from build123d import *

# Parameters (mm, degrees)
SKETCH1_W              = 22.27
SKETCH1_H              = 37
BOSS_EXTRUDE1_DEPTH    = 60
SHELL1_T               = -1
CONVERT_SOLID1_DEPTH   = 60
CONVERT_SOLID1_2_DEPTH = 60
SKETCH6_R              = 2.25
CUT_EXTRUDE1_DEPTH     = 72.365175156


# Read off the part's stored shape, not the designer's step: Convert-Solid1
with BuildPart() as part:
    # Sketch1 → Boss-Extrude1 (new body)
    with BuildSketch(Plane.XY):
        Rectangle(SKETCH1_W, SKETCH1_H)
    extrude(amount=BOSS_EXTRUDE1_DEPTH)

    # Shell1
    shell1_openings = [part.faces().sort_by_distance(p)[0] for p in [
        (0, 0, 60),
        (0, 0, 0),
        (11.135, 0, 30),
    ]]
    offset(amount=SHELL1_T, openings=shell1_openings, kind=Kind.INTERSECTION)

    # Convert-Solid1 outline → Convert-Solid1 (cut)
    with BuildSketch(Plane.XY):
        with BuildLine():
            Line((-11.135, 18.5), (-11.135, 16.23))
            ThreePointArc((-11.135, 16.23), (-10.470132393, 17.835132393), (-8.865, 18.5))
            Line((-8.865, 18.5), (-11.135, 18.5))
        make_face()
        with BuildLine():
            ThreePointArc((-8.865, -18.5), (-10.470132393, -17.835132393), (-11.135, -16.23))
            Line((-11.135, -16.23), (-11.135, -18.5))
            Line((-11.135, -18.5), (-8.865, -18.5))
        make_face()
    extrude(amount=CONVERT_SOLID1_DEPTH, mode=Mode.SUBTRACT)

    # Convert-Solid1 2 outline → Convert-Solid1 2 (add)
    with BuildSketch(Plane.XY):
        with BuildLine():
            Line((-10.135, 17.5), (-10.135, 16.23))
            ThreePointArc((-10.135, 16.23), (-9.763025612, 17.128025612), (-8.865, 17.5))
            Line((-8.865, 17.5), (-10.135, 17.5))
        make_face()
        with BuildLine():
            ThreePointArc((-8.865, -17.5), (-9.763025612, -17.128025612), (-10.135, -16.23))
            Line((-10.135, -16.23), (-10.135, -17.5))
            Line((-10.135, -17.5), (-8.865, -17.5))
        make_face()
    extrude(amount=CONVERT_SOLID1_2_DEPTH)

    # Sketch6 → Cut-Extrude1 (cut, through all)
    with BuildSketch(Plane(origin=(0, 18.5, 0), x_dir=(1, 0, 0), z_dir=(0, 1, 0))):
        with Locations(Location((1.135, -43.5, 0), (0, 0, 270))):
            Circle(SKETCH6_R)
        with Locations(Location((1.135, -54.5, 0), (0, 0, 270))):
            Circle(SKETCH6_R)
    extrude(amount=-CUT_EXTRUDE1_DEPTH, mode=Mode.SUBTRACT)


solid = part.part
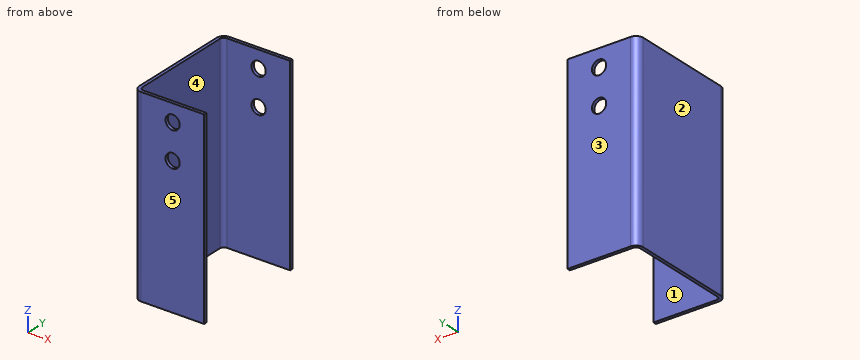
Work out the finished part from the listing and answer in its coordinate system (mm). Face numbers are marked on the shaded views. A direction names the side the tool comes from. Give positions to 0.01 mm unless a question says otherwise; leave off trailing zeros. Loops run counter-clockwise (first coordinate to the right, second up) from the corner with the lowest first, then second, coordinate; pieces in that order, holes last. Notation, with made-up numbers: (25.5, 52.5) -> (75.5, 52.5) arc R13 ccw to (75.5, 61.5) -> close; hole circle Ø11 at (59.25, 16.25). An arc over 180 degrees is marked (long way). Use a Markdown table: item, result. Add a question column.
1) This flat-tipped pin is pushed along its axis until it touches: P1, Ø5, axis at x = 1.135, z = 43.5, coming from the +Y side. Where does it stop, or does it pass through?
2) The part is cut by section C-C, the plane z = 11.5. Determine the outline of the cut face in (x, y) (3 decimals), plus the area to 3 significant figures.
3) For a pull along Y with two mould halves and no side action, classify the marked faces 3, 4 and 5 as +Y half, -Y half, draft (parallel to the pull), parting line (faces both ways), or undercut.
4) Consider line 1 along Y through (x, z) = (-3.25, 21); line 2 along X through (y, z) = (12, 42.5) (3 decimals); line 3 along X through (y, z) = (18.3, 54.5) (3 decimals). Determine where each line is inside the solid, lowest interval first.
5) The part is cut by section A-A, the plane x = -2.5. Determine the outline of the cut face in (y, z).
6) The part is cut by section B-B, the plane z = 54.5. Determine the outline of the cut face in (x, y) (3 decimals), plus the area to 3 significant figures.
7) Which of the six approach directions +Z, -Z, +X, -X, +Y, -Y give full straight-line access (tool end or side, diameter ignored) to the marked faces 1 and 2?
8) The part is cut by section D-D, the plane y = -7.5. Determine the outline of the cut face in (x, z) (3 decimals), plus the area to 3 significant figures.
Reported:
| question | item | result |
|---|---|---|
| 1 | P1 | stops at y = 18.5 |
| 2 | outline | (-11.135, -16.23) arc R2.27 ccw to (-8.865, -18.5) -> (11.135, -18.5) -> (11.135, -17.5) -> (-8.865, -17.5) arc R1.27 cw to (-10.135, -16.23) -> (-10.135, 16.23) arc R1.27 cw to (-8.865, 17.5) -> (11.135, 17.5) -> (11.135, 18.5) -> (-8.865, 18.5) arc R2.27 ccw to (-11.135, 16.23) -> close |
| 2 | area | 78.0 mm^2 |
| 3 | face 3 | +Y half |
| 3 | face 4 | undercut |
| 3 | face 5 | -Y half |
| 4 | line 1 | y = -18.5 to -17.5, 17.5 to 18.5 |
| 4 | line 2 | x = -11.135 to -10.135 |
| 4 | line 3 | x = -9.797 to -1.115, 3.385 to 11.135 |
| 5 | outline | (-18.5, 0) -> (-17.5, 0) -> (-17.5, 60) -> (-18.5, 60) -> close; (17.5, 0) -> (18.5, 0) -> (18.5, 60) -> (17.5, 60) -> close |
| 6 | outline | (-11.135, -16.23) arc R2.27 ccw to (-8.865, -18.5) -> (-1.115, -18.5) -> (-1.115, -17.5) -> (-8.865, -17.5) arc R1.27 cw to (-10.135, -16.23) -> (-10.135, 16.23) arc R1.27 cw to (-8.865, 17.5) -> (-1.115, 17.5) -> (-1.115, 18.5) -> (-8.865, 18.5) arc R2.27 ccw to (-11.135, 16.23) -> close; (3.385, -18.5) -> (11.135, -18.5) -> (11.135, -17.5) -> (3.385, -17.5) -> close; (3.385, 17.5) -> (11.135, 17.5) -> (11.135, 18.5) -> (3.385, 18.5) -> close |
| 6 | area | 69.0 mm^2 |
| 7 | face 1 | +Z, -Z, +X |
| 7 | face 2 | +Z, -Z, -X, +Y, -Y |
| 8 | outline | (-11.135, 0) -> (-10.135, 0) -> (-10.135, 60) -> (-11.135, 60) -> close |
| 8 | area | 60.0 mm^2 |
